Here's how the part is built. I have some questions about the finished solid (model axes, mm). Face numbers are marked on the shaded views. A direction names the side the tool comes from. Give positions to 0.01 mm unless a question says otherwise; leave off trailing zeros. Loops run counter-clockwise (first coordinate to the right, second up) from the corner with the lowest first, then second, coordinate; pieces in that order, holes last. Notation, with made-up numbers: (53.5, -12.75) - (84.5, -12.75) arc R32 ccw to (84.5, 21.25) - close; hole circle Ø5 at (60.25, -9.75). An arc over 180 degrees is marked (long way). Put each result on its own line as item: value. Start each with the question number.
from build123d import *

# Parameters (mm, degrees)
F0_W     = 6.35
F0_H     = 19.7729410879
F1_DEPTH = 25.4
F2_START = -12.7
F2_DEPTH = 12.7
F3_DEPTH = 12.7


with BuildPart() as f1:
    # F0 (on Right) → F1 (new body)
    with BuildSketch(Plane.YZ):
        with Locations((3.5528081138, -2.7100717787)):
            Rectangle(F0_W, F0_H)
    extrude(amount=-F1_DEPTH)

    # F0 (on Right) → F2 (join)
    with BuildSketch(Plane.YZ.offset(F2_START)):
        Polygon((-5.9721918862, 7.1763987653), (-18.6721918862, -12.5965423226), (0.3778081138, -12.5965423226), (0.3778081138, 7.1763987653), align=None)
    extrude(amount=-F2_DEPTH)

    # F0 (on Right) → F3 (join)
    with BuildSketch(Plane.YZ):
        Polygon((-18.6721918862, 0.1034576774), (-18.6721918862, -12.5965423226), (-5.9721918862, 7.1763987653), (0.3778081138, 7.1763987653), (6.7278081138, 7.1763987653), (6.7278081138, 12.8034576774), (-5.9721918862, 12.8034576774), align=None)
        with Locations((3.5528081138, -2.7100717787)):
            Rectangle(F0_W, F0_H)
        Polygon((-5.9721918862, 7.1763987653), (-18.6721918862, -12.5965423226), (0.3778081138, -12.5965423226), (0.3778081138, 7.1763987653), align=None)
    extrude(amount=F3_DEPTH)


solid = f1.part
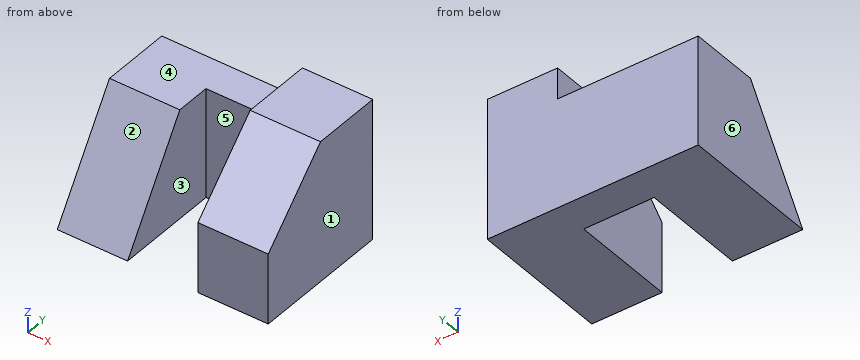
1) I need wall thicknesses on line 1 (X direction, y = -3, z = -6.5); line 2 (Y direction, x = -2, z = -4.5); line 3 (Z direction, x = -21, y = 3.75). Which ranges of each line are inside material? Lowest first, please.
2) Which directions (+Z, -Z, +X, -X, +Y, -Y) give clear straight access to the entire face, cutting with the end or side of a thin tool? Please do the marked faces 1, 2 and 3.
3) I'm going to push flat-ended pins straight in: P1, Ø3, axis at y = -4.5, z = 9.5, coming from the -X side; P2, Ø14, axis at x = -12.5, y = 2.5, coming from the +Z side. Where does each tip first touch, or does it pass through?
4) Thinking about a two-plate mould opening in X: for the marked faces 4, 5 and 6, which applies, pulls with the +X half, pulls with the -X half, needs draft (parallel to the pull), parting line crosses it, or undercut?
5) Suppose I cut it at C-C on z = -1.75. Please give me the cut outline in (x, y), plus the area to 3 significant figures.
6) Suppose I cut it at D-D on y = 2.25. Please give me the cut outline in (x, z).
7) Suppose I cut it at B-B on y = -16.25. Please give me the cut outline in (x, z), plus the area to 3 significant figures.
8) Suppose I cut it at A-A on x = 7. Please give me the cut outline in (y, z).
Ans:
1. line 1: x = -25.4 to -12.7, 0 to 12.7
1. line 2: y = 0.38 to 6.73
1. line 3: z = -12.6 to 7.18
2. face 1: +Z, -Z, +X, +Y, -Y
2. face 2: +Z, -X, -Y
2. face 3: +Z, -Z, -Y
3. P1: stops at x = 0
3. P2: stops at z = 7.18
4. face 4: needs draft
4. face 5: undercut
4. face 6: pulls with the -X half
5. outline: (-25.4, -11.71) - (-12.7, -11.71) - (-12.7, 0.38) - (0, 0.38) - (0, -18.67) - (12.7, -18.67) - (12.7, 6.73) - (-25.4, 6.73) - close
5. area: 637 mm²
6. outline: (-25.4, -12.6) - (12.7, -12.6) - (12.7, 12.8) - (0, 12.8) - (0, 7.18) - (-25.4, 7.18) - close
7. outline: (-25.4, -12.6) - (-12.7, -12.6) - (-12.7, -8.83) - (-25.4, -8.83) - close; (0, -12.6) - (12.7, -12.6) - (12.7, 2.53) - (0, 2.53) - close
7. area: 240 mm²
8. outline: (-18.67, -12.6) - (6.73, -12.6) - (6.73, 12.8) - (-5.97, 12.8) - (-18.67, 0.1) - close
